Can you work these out from the model? Positions are in its coordinate system, mm. A direction names the side the tool comes from. Give positions to 0.01 mm unless a question says otherwise; leave off trailing zeros. Write each loop counter-clockwise with the first axis right and the second up, starting at its lowest first coordinate (ties: lowest second). Pieces come first, ordered by that corner, then holes.
1. On a 3-axis mill with a long thin cutter (end or side, diameter ignored), from which of +Z, -Z, +X, -X, +Y, -Y can I reach the whole of each face in a straight line? I mean faces 1 (the flat face through (-1.89, -12.95, 121.56)), 2 (the flat face through (4, -12.4, 250)). Say none if no direction works.
2. Suppose I cut it at A-A (x = 0). Please give me the cut outline in (y, z).
3. Thinking about a two-plate mould opening in Y: for faces 3 (the flat face through (-3.4, -17.55, 122.9)), 4 (the cylindrical face through (-12.688, 0.558, 123.25)), 5 (the cylindrical face through (-0.81, -15.22, 121.34)), which applies, pulls with the +Y half, pulls with the -Y half, needs draft (parallel to the pull), parting line crosses it, or undercut?
4. Suppose I cut it at C-C (z = 125). Please give me the cut outline in (x, y), and give its area (3 significant figures).
5. I'm going to push flat-ended pins straight in: pin 1 (1.5 mm diameter, centred on x = -10.5, z = 68, fed in from -Y); pin 2 (4.5 mm diameter, centred on x = -0.5, z = 127.5, fed in from -Y); pin 3 (10 mm diameter, centred on x = 0, z = 125, fed in from +Y). Where does each tip first touch, or does it pass through?
6. If I drill on probe 1 along Z at (x, y) = (0, -14.65); probe 2 along Z at (x, y) = (0, 14.5); probe 3 along Y at (x, z) = (0.5, 154), over which ranges is the centre line in solid material (lowest first)?
7. Suppose I cut it at B-B (y = 0). Please give me the cut outline in (x, z).
8. Suppose I cut it at D-D (z = 204.5). Please give me the cut outline in (x, y).
```python
from build123d import *

# Parameters (mm, degrees)
F0_R      = 19.05
F0_R_2    = 12.7
F1_DEPTH  = 250
F2_R      = 3.75
F3_DEPTH  = 19.051
F4_DEPTH  = 19.051
F6_R      = 8
F7_DEPTH  = 32
F9_R      = 10
F10_DEPTH = 1.5


with BuildPart() as f1:
    # F0 (on Top) → F1 (new body)
    with BuildSketch(Plane.XY):
        Circle(F0_R)
        Circle(F0_R_2, mode=Mode.SUBTRACT)
    extrude(amount=F1_DEPTH)

    # F2 (on Front) → F3 (cut, through all)
    with BuildSketch(Plane.XZ):
        with Locations((0, 125)):
            Circle(F2_R)
    extrude(amount=-F3_DEPTH, mode=Mode.SUBTRACT)

    # F2 (on Front) → F4 (cut, through all)
    with BuildSketch(Plane.XZ):
        with Locations((0, 125)):
            Circle(F2_R)
    extrude(amount=F4_DEPTH, mode=Mode.SUBTRACT)

    # F6 (on offset) → F7 (cut)
    with BuildSketch(Plane.XZ.offset(-19.05)):
        with Locations((0, 125)):
            Circle(F6_R)
    extrude(amount=F7_DEPTH, mode=Mode.SUBTRACT)

    # F9 (on offset) → F10 (cut)
    with BuildSketch(Plane.XZ.offset(19.05)):
        with Locations((0, 125)):
            Circle(F9_R)
    extrude(amount=-F10_DEPTH, mode=Mode.SUBTRACT)


solid = f1.part
```
Checks:
1. face 1: +Y
1. face 2: +Z, +X, -X, +Y, -Y
2. outline: (-19.05, 0) - (-12.7, 0) - (-12.7, 117) - (-12.95, 117) - (-12.95, 121.25) - (-17.55, 121.25) - (-17.55, 115) - (-19.05, 115) - close; (-19.05, 135) - (-17.55, 135) - (-17.55, 128.75) - (-12.95, 128.75) - (-12.95, 133) - (-12.7, 133) - (-12.7, 250) - (-19.05, 250) - close; (12.7, 0) - (19.05, 0) - (19.05, 117) - (12.7, 117) - close; (12.7, 133) - (19.05, 133) - (19.05, 250) - (12.7, 250) - close
3. face 3: pulls with the -Y half
3. face 4: undercut
3. face 5: needs draft
4. outline: (-8, -12.95) - (-8, -9.86) arc R12.7 cw to (-8, 9.86) - (-8, 17.29) arc R19.05 ccw to (-7.41, -17.55) - (-3.75, -17.55) - (-3.75, -12.95) - close; (3.75, -17.55) - (7.41, -17.55) arc R19.05 ccw to (8, 17.29) - (8, 9.86) arc R12.7 cw to (8, -9.86) - (8, -12.95) - (3.75, -12.95) - close
4. area: 459 mm2
5. pin 1: stops at y = -16.37
5. pin 2: stops at y = -17.55
5. pin 3: stops at y = -12.95
6. probe 1: z = 0 to 121.25, 128.75 to 250
6. probe 2: z = 0 to 117, 133 to 250
6. probe 3: y = -19.04 to -12.69, 12.69 to 19.04
7. outline: (-19.05, 0) - (-12.7, 0) - (-12.7, 250) - (-19.05, 250) - close; (12.7, 0) - (19.05, 0) - (19.05, 250) - (12.7, 250) - close
8. outline: circle Ø38.1 at (0, 0); hole circle Ø25.4 at (0, 0)
